Job drawing, mm, ordinate dimensions from the low corner. One solid piece. A direction names the side the tool comes from. Give positions to 0.01 mm unless a question says otherwise; leave off trailing zeros. Order: outer loops, then holes, each group sorted by start corner. A loop starts at its lowest first (then second) coordinate and runs counter-clockwise, first axis right, second up.
Item 1: Wall check: L1, parallel to X at y = 229, z = 528.5; L2, parallel to Y at x = 466, z = 509.5. Give the ranges that are in metal, low to high.
Item 2: Flat gauge pins, fed straight in: P1, Ø12.5, axis at y = 619, z = 152.5, coming from the +X side; P2, Ø8, axis at x = 18.5, z = 524.5, coming from the -Y side; P3, Ø10, axis at x = 402, z = 154.5, coming from the -Y side. Where does each tip first touch, or does it go through?
Item 3: Band-saw the part on B-B on x = 372. Give the cut face in (y, z) (1 decimal), plus the area to 3 significant figures.
Item 4: Band-saw the part on A-A on y = 596. Give the cut face in (x, z) (1 decimal).
Item 5: Which spindle directions (+Z, -Z, +X, -X, +Y, -Y) get a long thin tool onto all of the face, cutting with end or side? Do the marked faces 1 and 2. Say none if no direction does.
Item 6: Band-saw the part on C-C on z = 420. Give the cut face in (x, y), plus the area to 3 significant figures.
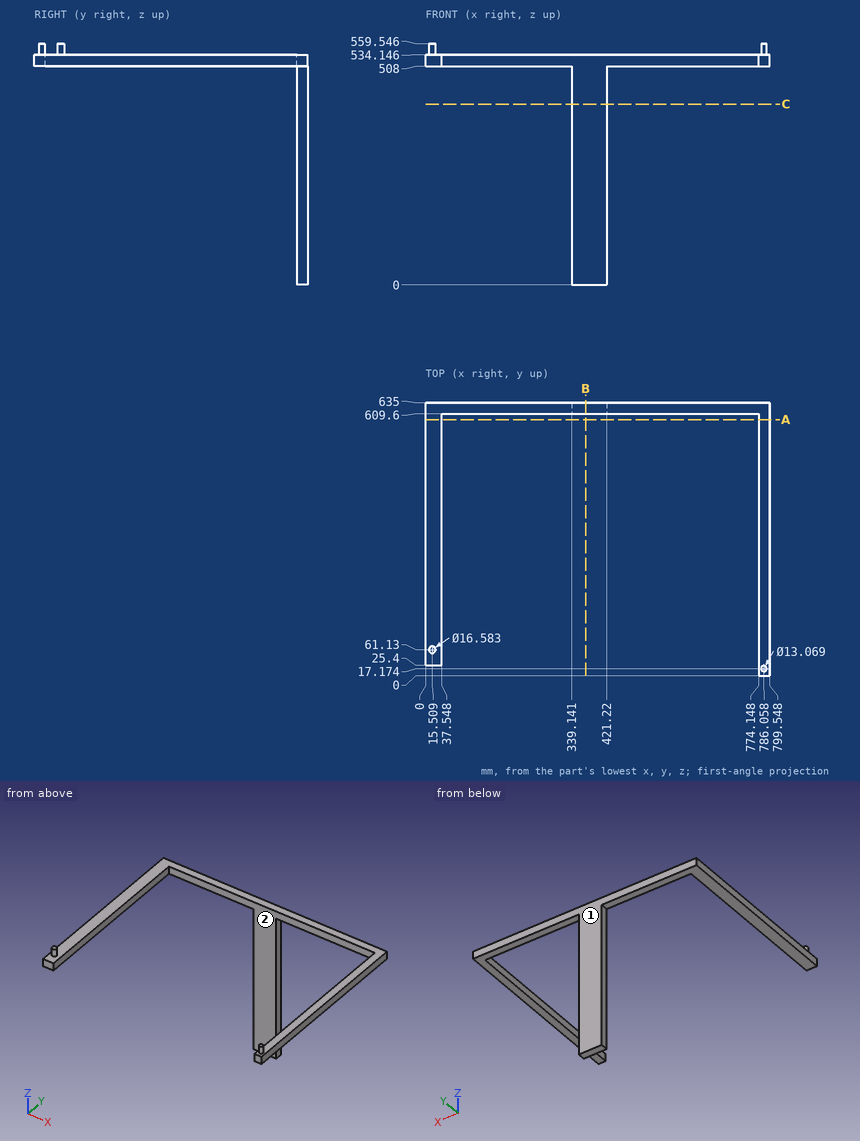
The answers:
1. L1: x = 0 to 37.55, 774.15 to 799.55
1. L2: y = 609.6 to 635
2. P1: stops at x = 421.22
2. P2: stops at y = 25.4
2. P3: stops at y = 609.6
3. outline: (609.6, 0) - (635, 0) - (635, 534.1) - (609.6, 534.1) - close
3. area: 13,600 mm2
4. outline: (0, 508) - (37.5, 508) - (37.5, 534.1) - (0, 534.1) - close; (774.1, 508) - (799.5, 508) - (799.5, 534.1) - (774.1, 534.1) - close
5. face 1: +Z, -Z, +X, -X, +Y
5. face 2: +Z, -Z, -Y
6. outline: (339.14, 609.6) - (421.22, 609.6) - (421.22, 635) - (339.14, 635) - close
6. area: 2,080 mm2
